Part print with two shaded views. Sizes in mm from the minimum x, y, z corner. A direction names the side the tool comes from. Round coordinates to 2 decimals unless told otherwise and drop trailing zeros. Write each loop counter-clockwise with the first axis right and the second up, starting at its lowest first coordinate (ties: lowest second). Pieces come first, ordered by that corner, then holes. Notation, with made-up numbers: (9, 52) -> (55, 52) arc R16 cw to (55, 69) -> close; hole circle Ø6 at (55.5, 7.25). An arc over 180 degrees is marked (long way). Return JSON: item names as keys, results as strings.
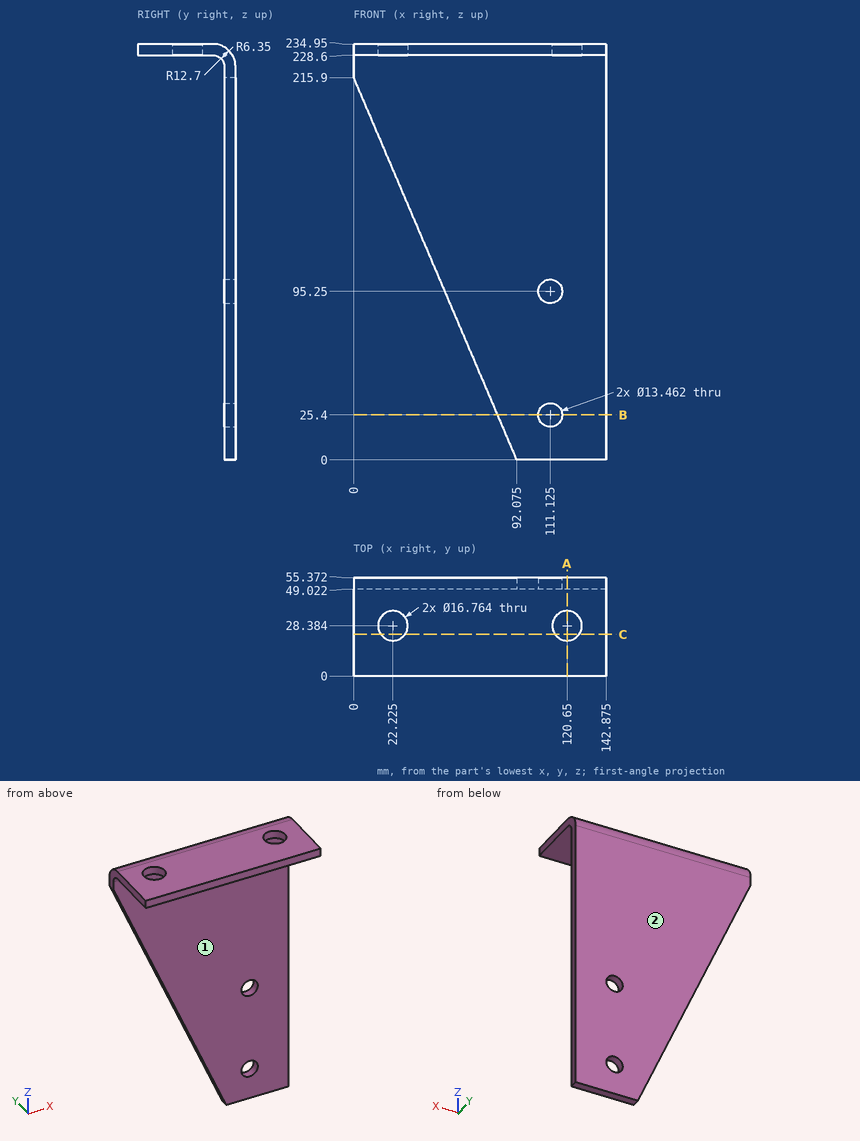
Q1. Saw through at C-C on y = 23.5. Count the separate pieces of the cut face and the enclosed holes in it.
Verdict:
{"separate pieces": "3", "enclosed holes": "0"}
Q2. Saw through at A-A on x = 120.65. List the corners of the cut face in (y, z), then the cut area to 3 significant figures.
Verdict:
{"outline": "(0, 228.6) -> (20, 228.6) -> (20, 234.95) -> (0, 234.95) -> close; (36.77, 228.6) -> (42.67, 228.6) arc R6.35 cw to (49.02, 222.25) -> (49.02, 0) -> (55.37, 0) -> (55.37, 222.25) arc R12.7 ccw to (42.67, 234.95) -> (36.77, 234.95) -> close", "area": "1,670 mm²"}
Q3. Saw through at B-B on z = 25.4. List the corners of the cut face in (x, y) (1 decimal), then the cut area to 3 significant figures.
Verdict:
{"outline": "(81.2, 49) -> (104.4, 49) -> (104.4, 55.4) -> (81.2, 55.4) -> close; (117.9, 49) -> (142.9, 49) -> (142.9, 55.4) -> (117.9, 55.4) -> close", "area": "306 mm²"}
Q4. Wall check: L1, parallel to Z at x = 112.5, y = 31; L2, parallel to Y at x = 111, z = 46; L3, parallel to Z at x = 76, y = 43 (1 decimal). Give the ranges that are in metal, low to high.
Verdict:
{"L1": "z = 228.6 to 234.95", "L2": "y = 49.02 to 55.37", "L3": "z = 228.6 to 234.9"}
Q5. 3-axis set-ups, long thin cutter, end or side, ignore diameter. For the marked faces 1 and 2: which of +Z, -Z, +X, -X, +Y, -Y reach the whole face in a straight line?
Verdict:
{"face 1": "-Z, +X, -X, -Y", "face 2": "+Z, -Z, +X, -X, +Y"}
Q6. Pin check, flat tips, straight feed: pin 1 Ø15 at (x, y) = (120.65, 28.38) entering from -Z; pin 2 Ø6 at (x, z) = (94.5, 98.5) entering from -Y; pin 3 Ø3 at (x, y) = (55.5, 28) entering from -Z. Stop position of each tip, or through.
Verdict:
{"pin 1": "passes through", "pin 2": "stops at y = 49.02", "pin 3": "stops at z = 228.6"}
